Can you work these out from the model? Positions are in its coordinate system, mm. Round coordinates to 2 decimals unless told otherwise and drop trailing zeros. Order: outer loops, then holes, each group sorted by start corner. A loop starts at its lowest first (then second) coordinate and runs counter-clockwise, first axis right, second up.
Q1. Will these pins go through, and if not, where does the flat tip stop? P1, Ø3.5, axis at x = 3, z = -19, coming from the +Y side; P2, Ø1.1, axis at x = 7, z = -16.5, coming from the +Y side.
Q2. If we section it at A-A (z = -5): Please give me the cut outline in (x, y), plus the area to 3 significant figures.
Q3. If we section it at B-B (x = 3): Please give me the cut outline in (y, z), plus the area to 3 significant figures.
Q4. If I drill on line 1 (X direction, y = 0.7, z = -19); line 2 (X direction, y = 0.45, z = -19); line 3 (Y direction, x = 2.25, z = -16.25), over which ranges is the centre line in solid material (lowest first)?
Q5. If we section it at C-C (z = -7.75): Please give me the cut outline in (x, y).
Q6. If we section it at D-D (x = 7): Please give me the cut outline in (y, z).
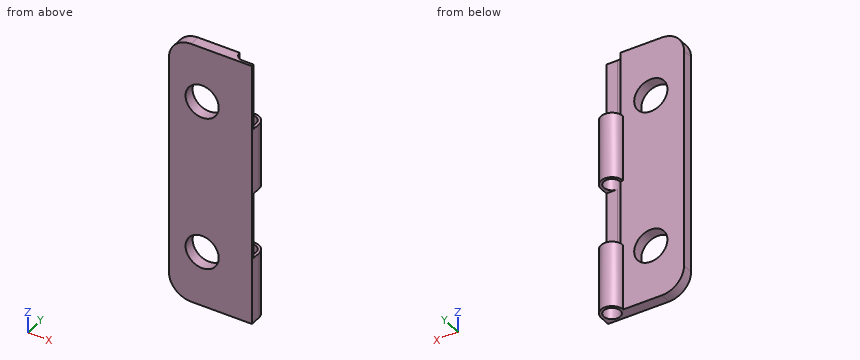
from build123d import *

# Parameters (mm, degrees)
CROQUIS1_W              = 7.5
CROQUIS1_H              = 24
SALIENTE_EXTRUIR1_DEPTH = 1
CROQUIS2_R              = 1
SALIENTE_EXTRUIR2_DEPTH = 6
CROQUIS3_R              = 1
SALIENTE_EXTRUIR3_DEPTH = 6
CROQUIS4_R              = 0.75
CORTAR_EXTRUIR1_DEPTH   = 24
REDONDEO1_R             = 2
CROQUIS5_R              = 1.5
CORTAR_EXTRUIR2_DEPTH   = 18
CORTAR_EXTRUIR3_DEPTH   = 6
CORTAR_EXTRUIR4_DEPTH   = 6


with BuildPart() as part:
    # Croquis1 → Saliente-Extruir1 (new body)
    with BuildSketch(Plane(origin=(0, 0, 0), x_dir=(1, 0, 0), z_dir=(0, 1, 0))):
        with Locations((3.75, 12)):
            Rectangle(CROQUIS1_W, CROQUIS1_H)
    extrude(amount=SALIENTE_EXTRUIR1_DEPTH)

    # Croquis2 → Saliente-Extruir2 (add)
    with BuildSketch(Plane(origin=(0, 0, -24), x_dir=(-1, 0, 0), z_dir=(0, 0, -1))):
        with Locations((-6.5, 1)):
            Circle(CROQUIS2_R)
    extrude(amount=-SALIENTE_EXTRUIR2_DEPTH)

    # Croquis3 → Saliente-Extruir3 (add)
    with BuildSketch(Plane.XY.offset(-12)):
        with Locations((6.5, 1)):
            Circle(CROQUIS3_R)
    extrude(amount=SALIENTE_EXTRUIR3_DEPTH)

    # Croquis4 → Cortar-Extruir1 (cut)
    with BuildSketch(Plane(origin=(0, 0, -24), x_dir=(-1, 0, 0), z_dir=(0, 0, -1))):
        with Locations((-6.5, 1)):
            Circle(CROQUIS4_R)
    extrude(amount=-CORTAR_EXTRUIR1_DEPTH, mode=Mode.SUBTRACT)

    # Redondeo1
    redondeo1_edges = [part.edges().sort_by_distance(p)[0] for p in [
        (0, 0.5, -24),
        (0, 0.5, 0),
    ]]
    fillet(redondeo1_edges, radius=REDONDEO1_R)

    # Croquis5 → Cortar-Extruir2 (cut)
    with BuildSketch(Plane(origin=(0, 1, 0), x_dir=(1, 0, 0), z_dir=(0, 1, 0))):
        with Locations(Location((3, 19, 0), (0, 0, 270))):
            Circle(CROQUIS5_R)
        with Locations(Location((3, 5, 0), (0, 0, 270))):
            Circle(CROQUIS5_R)
    extrude(amount=-CORTAR_EXTRUIR2_DEPTH, mode=Mode.SUBTRACT)

    # Croquis6 → Cortar-Extruir3 (cut)
    with BuildSketch(Plane.XY):
        Polygon((6.5, 0.25), (7.5, 0.25), (7.5, 1), (7.25, 1), align=None)
    extrude(amount=-CORTAR_EXTRUIR3_DEPTH, mode=Mode.SUBTRACT)

    # Croquis7 → Cortar-Extruir4 (cut)
    with BuildSketch(Plane(origin=(0, 0, -12), x_dir=(-1, 0, 0), z_dir=(0, 0, -1))):
        Polygon((-6.5, 0.25), (-7.5, 0.25), (-7.5, 1), (-6.800248099, 1), align=None)
    extrude(amount=CORTAR_EXTRUIR4_DEPTH, mode=Mode.SUBTRACT)


solid = part.part
Solution:
1. P1: stops at y = 1
1. P2: stops at y = 0.25
2. outline: (0, 0) - (1.5, 0) - (1.5, 1) - (0, 1) - close; (4.5, 0) - (7.5, 0) - (7.5, 0.25) - (6.5, 0.25) arc R0.75 cw to (5.75, 1) - (4.5, 1) - close
2. area: 3.31 mm2
3. outline: (0, -24) - (1, -24) - (1, -20.5) - (0, -20.5) - close; (0, -17.5) - (1, -17.5) - (1, -6.5) - (0, -6.5) - close; (0, -3.5) - (1, -3.5) - (1, 0) - (0, 0) - close
3. area: 18.0 mm2
4. line 1: x = 0 to 1.5, 4.5 to 5.81, 7.19 to 7.5
4. line 2: x = 0 to 1.5, 4.5 to 5.99, 7.01 to 7.5
4. line 3: y = 0 to 1
5. outline: (0, 0) - (7.5, 0) - (7.5, 1) arc R1 ccw to (5.5, 1) - (0, 1) - close; hole circle Ø1.5 at (6.5, 1)
6. outline: (0, -24) - (0.44, -24) - (0.44, -18) - (0.25, -18) - (0.25, -12) - (0.44, -12) - (0.44, -6) - (0.25, -6) - (0.25, 0) - (0, 0) - close; (1.56, -24) - (1.87, -24) - (1.87, -18) - (1.56, -18) - close; (1.56, -12) - (1.87, -12) - (1.87, -6) - (1.56, -6) - close
